from build123d import *

# Parameters (mm, degrees)
F0_R     = 1.6
F0_R_2   = 2
F1_DEPTH = 7
F2_R     = 2
F3_DEPTH = 25
F4_COUNT = 4
F7_DEPTH = 6
F8_SIZE  = 0.5


with BuildPart() as f1:
    # F0 (on Front) → F1 (new body)
    with BuildSketch(Plane.XZ):
        with BuildLine():
            Line((-9.192388, -1.414214), (-1.414214, -9.192388))
            ThreePointArc((-1.414214, -9.192388), (0, -9.778175), (1.414214, -9.192388))
            Line((1.414214, -9.192388), (9.192388, -1.414214))
            ThreePointArc((9.192388, -1.414214), (9.778175, 0), (9.192388, 1.414214))
            Line((9.192388, 1.414214), (1.414214, 9.192388))
            ThreePointArc((1.414214, 9.192388), (0, 9.778175), (-1.414214, 9.192388))
            Line((-1.414214, 9.192388), (-9.192388, 1.414214))
            ThreePointArc((-9.192388, 1.414214), (-9.778175, 0), (-9.192388, -1.414214))
        make_face()
        with Locations((0, -7)):
            Circle(F0_R, mode=Mode.SUBTRACT)
        with Locations((-7, 0)):
            Circle(F0_R, mode=Mode.SUBTRACT)
        Circle(F0_R_2, mode=Mode.SUBTRACT)
        with Locations((7, 0)):
            Circle(F0_R, mode=Mode.SUBTRACT)
        with Locations((0, 7)):
            Circle(F0_R, mode=Mode.SUBTRACT)
    extrude(amount=F1_DEPTH)


with BuildPart() as f3:
    # F2 (on face) → F3 (new body)
    with BuildSketch(Plane(origin=(-5.303301, 0, -5.303301), x_dir=(0.707107, 0, -0.707107), z_dir=(-0.707107, 0, -0.707107))):
        with Locations((0, 4)):
            Circle(F2_R)
    extrude(amount=-F3_DEPTH)


with BuildPart() as f4_1:
    # F4: instance of F3
    add(f3.part.rotate(Axis((0, 0, 0), (0, 1, 0)), 1 * 360 / F4_COUNT))


with BuildPart() as f4_2:
    # F4: instance of F3
    add(f3.part.rotate(Axis((0, 0, 0), (0, 1, 0)), 2 * 360 / F4_COUNT))


with BuildPart() as f4_3:
    # F4: instance of F3
    add(f3.part.rotate(Axis((0, 0, 0), (0, 1, 0)), 3 * 360 / F4_COUNT))


with BuildPart() as f1_1:
    add(f1.part)

    # F5: cut F3, F4_1, F4_2, F4_3
    add(f3.part, mode=Mode.SUBTRACT)
    add(f4_1.part, mode=Mode.SUBTRACT)
    add(f4_2.part, mode=Mode.SUBTRACT)
    add(f4_3.part, mode=Mode.SUBTRACT)

    # F6 (on face) → F7 (cut)
    with BuildSketch(Plane.XZ.offset(7)):
        Polygon((-1.449569, 5.338656), (-3.394113, 3.394113), (-5.338656, 1.449569), (-3.570889, -0.318198), (0.318198, 3.570889), align=None)
    extrude(amount=-F7_DEPTH, mode=Mode.SUBTRACT)

    # F8
    f8_edges = [f1_1.edges().sort_by_distance(p)[0] for p in [
        (5.4, 0, 0),
        (-1.6, 0, 7),
        (-8.6, 0, 0),
        (-1.6, 0, -7),
    ]]
    chamfer(f8_edges, length=F8_SIZE)


solid = f1_1.part
For this review, take the finished solid that the model builds, in its own axes (mm). Coordinates: 2 decimals unless noted, no trailing zeros. Loops run counter-clockwise (first coordinate to the right, second up) from the corner with the lowest first, then second, coordinate; pieces in that order, holes last. Notation, with made-up numbers: (86.5, -19) - (111.5, -19) arc R17 cw to (111.5, -14) - close; hole circle Ø2 at (74.5, 42). An arc over 180 degrees is marked (long way). Return JSON: item names as keys, results as strings.
Item 1: Take a section at A-A (y = -6.5). Give the boundary of the cut face in (x, z).
Determined:
{"outline": "(-9.19, -1.41) - (-1.41, -9.19) arc R2 ccw to (1.41, -9.19) - (9.19, -1.41) arc R2 ccw to (9.19, 1.41) - (1.41, 9.19) arc R2 ccw to (-1.41, 9.19) - (-9.19, 1.41) arc R2 ccw to start; hole circle Ø3.2 at (-7, 0); hole (-5.34, 1.45) - (-3.57, -0.32) - (0.32, 3.57) - (-1.45, 5.34) - (-3.39, 3.39) - close; hole circle Ø4 at (0, 0); hole circle Ø3.2 at (0, -7); hole circle Ø3.2 at (0, 7); hole circle Ø3.2 at (7, 0)"}
Item 2: For line 1 (Z direction, x = 0, y = -1.5); line 2 (X direction, y = -6.5, z = 1.25); line 3 (X direction, y = -4.5, z = -1.25), list the stretches that pass through material, from the lowest coordinate up.
Determined:
{"line 1": "z = -9.78 to -8.6, -5.4 to -2, 2 to 3.25, 3.89 to 5.4, 8.6 to 9.78", "line 2": "x = -9.34 to -8, -6 to -5.14, -2 to -1.56, 1.56 to 6, 8 to 9.34", "line 3": "x = -9.34 to -8, -6 to -3.99, 3.99 to 6, 8 to 9.34"}
Item 3: Insertion check: pin 1 (3 mm diameter, centred on x = 0, z = 0, fed in from -Y); pin 2 (3.5 mm diameter, centred on x = 0, z = 7, fed in from +Y); pin 3 (4 mm diameter, centred on x = 6, y = -2.5, fed in from -Z). Each pin has a flat end and moves straight along its axis. Give the tip position at first contact, or say it passes through.
Determined:
{"pin 1": "passes through", "pin 2": "stops at y = -0.35", "pin 3": "stops at z = -6.61"}
Item 4: Take a section at B-B (y = -0.25). Give the boundary of the cut face in (x, z).
Determined:
{"outline": "(-9.19, -1.41) - (-1.41, -9.19) arc R2 ccw to (1.41, -9.19) - (9.19, -1.41) arc R2 ccw to (9.19, 1.41) - (1.41, 9.19) arc R2 ccw to (-1.41, 9.19) - (-9.19, 1.41) arc R2 ccw to start; hole circle Ø3.7 at (-7, 0); hole circle Ø4 at (0, 0); hole circle Ø3.7 at (0, -7); hole circle Ø3.7 at (0, 7); hole circle Ø3.7 at (7, 0)"}
Item 5: Mouldability with a two-part tool opening along X and no side actions: class faces 1 (the cylindrical face through (-9.78, -3.45, 0.02)), 2 (the cylindrical face through (-0.02, -3.45, -9.78)), 3 (the flat face through (2, 0, -2)), 4 (the flat face through (-3, -1, 3)) as pulls with the +X half, pulls with the -X half, needs draft (parallel to the pull), parting line crosses it, or undercut.
Determined:
{"face 1": "pulls with the -X half", "face 2": "parting line crosses it", "face 3": "needs draft", "face 4": "undercut"}
Item 6: Take a section at C-C (x = 7). Give the boundary of the cut face in (y, z), then the cut area to 3 significant figures.
Determined:
{"outline": "(-7, -3.61) - (0, -3.61) - (0, -2.1) - (-0.5, -1.6) - (-7, -1.6) - close; (-7, 1.6) - (-0.5, 1.6) - (0, 2.1) - (0, 3.61) - (-7, 3.61) - close", "area": "27.8 mm2"}
Item 7: Take a section at D-D (z = 7). Give the boundary of the cut face in (x, y), then the cut area to 3 significant figures.
Determined:
{"outline": "(-3.61, -7) - (-1.6, -7) - (-1.6, -0.5) - (-2.1, 0) - (-3.61, 0) - close; (1.6, -7) - (3.61, -7) - (3.61, 0) - (2.1, 0) - (1.6, -0.5) - close", "area": "27.8 mm2"}
